Part model, mm, in its own coordinate system. A direction names the side the tool comes from. Give positions to 0.01 mm unless a question says otherwise; leave off trailing zeros. Order: outer loops, then holes, each group sorted by start corner. A loop starts at its lowest first (then second) coordinate and runs counter-clockwise, first axis right, second up.
1. Drop a flat-ended pin along its axis: pin 1 Ø12 at (x, z) = (-23.5, -13) entering from -Y. Give the stop position or say it passes through.
2. Slice it at C-C on z = 45.5. List the corners of the cut face in (x, y), and give its area (3 significant figures).
3. Slice it at A-A on y = -30. Give the number of separate pieces and of enclosed holes in the cut face, and give its area (3 significant figures).
4. Which spindle directions (+Z, -Z, +X, -X, +Y, -Y) get a long thin tool onto all of the face, cutting with end or side? Do faces 1 (the flat face through (-141.936, -19, 114)), 2 (the flat face through (-174.304, -19, -3)), 3 (the flat face through (-37, -20, -238.579)). Say none if no direction does.
5. Probe line 1 (Z direction, x = -104, y = -1.5); line 2 (X direction, y = -21, z = -128.5); line 3 (X direction, y = -20, z = 204). List the from-to ranges inside material, lowest first.
6. Mould opens along Z. For faces 4 (the flat face through (-144.476, -20, 114)), 5 (the flat face through (79.933, -20, 155)), 6 (the flat face through (105.096, -19, -3)), 7 (the flat face through (-37, -19, -241.119)) say: +Z half, -Z half, draft (parallel to the pull), parting line (faces both ways), or undercut.
from build123d import *

# Parameters (mm, degrees)
F0_W     = 279.4
F0_H     = 482.6
F0_W_2   = 218.44
F0_H_2   = 25.4
F1_DEPTH = 38.1
F2_DEPTH = 25.4
F3_T     = -2.54


with BuildPart() as f1:
    # F0 (on Front) → F1 (new body)
    with BuildSketch(Plane.XZ):
        with Locations((-34.6037362662, 0.1808144152)):
            Rectangle(F0_W, F0_H)
        with Locations((-32.7158253479, 113.7473966599)):
            Rectangle(F0_W_2, F0_H_2, mode=Mode.SUBTRACT)
        with Locations((-31.8270157862, 155.5219079971)):
            Rectangle(F0_W_2, F0_H_2, mode=Mode.SUBTRACT)
        with Locations((-32.7158253479, 202.6293214083)):
            Rectangle(F0_W_2, F0_H_2, mode=Mode.SUBTRACT)
    extrude(amount=F1_DEPTH)

    # F0 (on Front) → F2 (join)
    with BuildSketch(Plane.XZ):
        with Locations((-34.6037362662, 0.1808144152)):
            Rectangle(F0_W, F0_H)
        with Locations((-32.7158253479, 113.7473966599)):
            Rectangle(F0_W_2, F0_H_2, mode=Mode.SUBTRACT)
        with Locations((-31.8270157862, 155.5219079971)):
            Rectangle(F0_W_2, F0_H_2, mode=Mode.SUBTRACT)
        with Locations((-32.7158253479, 202.6293214083)):
            Rectangle(F0_W_2, F0_H_2, mode=Mode.SUBTRACT)
    extrude(amount=F2_DEPTH)

    # F3
    f3_openings = [f1.faces().sort_by_distance(p)[0] for p in [
        (-34.911334, -38.1, -21.946168),
    ]]
    offset(amount=F3_T, openings=f3_openings, kind=Kind.INTERSECTION)


solid = f1.part
Data:
1. pin 1: stops at y = -2.54
2. outline: (-174.3, -38.1) - (-171.76, -38.1) - (-171.76, -2.54) - (102.56, -2.54) - (102.56, -38.1) - (105.1, -38.1) - (105.1, 0) - (-174.3, 0) - close
2. area: 890 mm2
3. separate pieces: 4
3. enclosed holes: 4
3. area: 7,640 mm2
4. face 1: +Y, -Y
4. face 2: +Z, -Z, -X, +Y, -Y
4. face 3: -Y
5. line 1: z = -241.12 to 101.05, 126.45 to 142.82, 168.22 to 189.93, 215.33 to 241.48
5. line 2: x = -174.3 to -171.76, 102.56 to 105.1
5. line 3: x = -174.3 to -171.76, -144.48 to -141.94, 76.5 to 79.04, 102.56 to 105.1
6. face 4: undercut
6. face 5: undercut
6. face 6: draft
6. face 7: -Z half
